The listing builds one solid part. Answer for the finished solid, in the listing's coordinates (mm). Coordinates: 2 decimals unless noted, no trailing zeros. Order: outer loops, then holes, each group sorted by start corner. A loop starts at its lowest first (then second) coordinate and runs counter-clockwise, first axis right, second up. Notation, with made-up numbers: (-15, 53.5) - (3, 53.5) arc R31 ccw to (3, 78.5) - close; hole circle Ø11 at (36.25, -15). An arc over 180 degrees is marked (long way). Use one line per item in the form item = value. Start each with the question number.
Item 1: Consider line 1 along Z through (x, y) = (-75, 3.5); line 2 along Z through (x, y) = (-76.5, 4.25); line 3 along Y through (x, z) = (-68.5, 33.5). Determine where each line is inside the solid, lowest interval first. Write a range as [from, to].
Item 2: Each of these flat-tipped pins is pushed along its axis until it touches: pin 1 Ø5 at (x, z) = (-81, 8.5) entering from +Y; pin 2 Ø4 at (x, z) = (-75, 30) entering from +Y; pin 3 Ø1.5 at (y, z) = (15, 31) entering from -X. Where does it stop, or does it pass through?
Item 3: Section A-A, the plane y = 7.5 is taken. Write down the section's boundary in (x, z), and give its area (3 significant figures).
Item 4: Section B-B, the plane z = 35.5 is taken. Write down the section's boundary in (x, y).
Item 5: Section C-C, the plane z = 23 is taken. Write down the section's boundary in (x, y).
Item 6: Section D-D, the plane x = -78.5 is taken. Write down the section's boundary in (y, z), and give its area (3 significant figures).
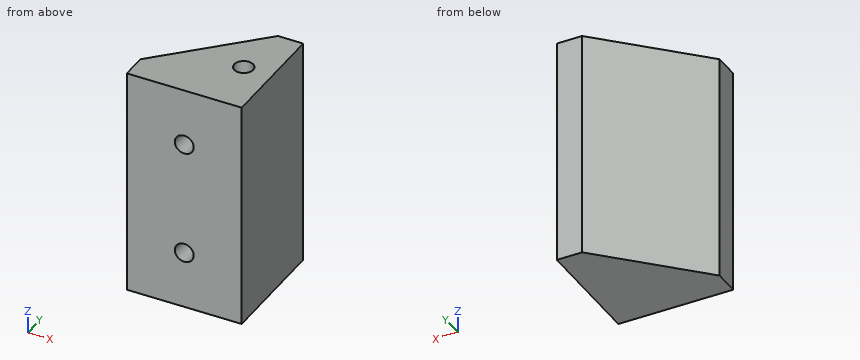
from build123d import *

# Parameters (mm, degrees)
PAD_DEPTH      = 40
SKETCH001_R    = 1.65
HOLE_DEPTH     = 8
HOLE_TIPS_R    = 1.65
SKETCH002_R    = 1.65
HOLE001_DEPTH  = 8
HOLE001_TIPS_R = 1.65


with BuildPart() as part:
    # Sketch → Pad (new body)
    with BuildSketch(Plane.XY):
        Polygon((-85, 0), (-65, 0), (-65, 20), (-69.4, 20), (-85, 4.4), align=None)
    extrude(amount=PAD_DEPTH)

    # Sketch001 (on Face1 of Pad) → Hole (cut)
    with BuildSketch(Plane.XZ):
        with Locations((-75, 30)):
            Circle(SKETCH001_R)
        with Locations((-75, 10)):
            Circle(SKETCH001_R)
    extrude(amount=-HOLE_DEPTH, mode=Mode.SUBTRACT)

    # Hole tips → Hole tip 1 section 0
    with BuildSketch(Plane.XZ.offset(-8), mode=Mode.PRIVATE) as hole_tip_1_s0:
        with Locations((-75, 30)):
            Circle(HOLE_TIPS_R)
    loft([hole_tip_1_s0.sketch, Vertex(-75, 8.99142, 30)], mode=Mode.SUBTRACT)

    # Hole tips → Hole tip 2 section 0
    with BuildSketch(Plane.XZ.offset(-8), mode=Mode.PRIVATE) as hole_tip_2_s0:
        with Locations((-75, 10)):
            Circle(HOLE_TIPS_R)
    loft([hole_tip_2_s0.sketch, Vertex(-75, 8.99142, 10)], mode=Mode.SUBTRACT)

    # Sketch002 (on Face4 of Hole) → Hole001 (cut)
    with BuildSketch(Plane.XY.offset(40)):
        with Locations((-70, 10)):
            Circle(SKETCH002_R)
    extrude(amount=-HOLE001_DEPTH, mode=Mode.SUBTRACT)

    # Hole001 tips → Hole001 tip 1 section 0
    with BuildSketch(Plane.XY.offset(32), mode=Mode.PRIVATE) as hole001_tip_1_s0:
        with Locations((-70, 10)):
            Circle(HOLE001_TIPS_R)
    loft([hole001_tip_1_s0.sketch, Vertex(-70, 10, 31.00858)], mode=Mode.SUBTRACT)


solid = part.part
Response:
q1.line_1 = [0, 8.35], [11.65, 28.35], [31.65, 40]
q1.line_2 = [0, 9.31], [10.69, 29.31], [30.69, 40]
q1.line_3 = [0, 9.31], [10.69, 20]
q2.pin_1 = 10.9
q2.pin_2 = 16.4
q2.pin_3 = -75.15
q3.outline = (-81.9, 0) - (-65, 0) - (-65, 40) - (-81.9, 40) - close; hole circle Ø3.3 at (-75, 10); hole circle Ø3.3 at (-75, 30)
q3.area = 659 mm2
q4.outline = (-85, 0) - (-65, 0) - (-65, 20) - (-69.4, 20) - (-85, 4.4) - close; hole circle Ø3.3 at (-70, 10)
q5.outline = (-85, 0) - (-65, 0) - (-65, 20) - (-69.4, 20) - (-85, 4.4) - close
q6.outline = (0, 0) - (10.9, 0) - (10.9, 40) - (0, 40) - close
q6.area = 436 mm2
